Drawing for the job (mm, zero at the part's lowest x, y, z). A direction names the side the tool comes from. Coordinates: 2 decimals unless noted, no trailing zeros. Write each loop counter-clockwise with the first axis right and the second up, starting at its lowest first coordinate (ties: lowest second). Pieces come first, ordered by that corner, then holes. Notation, with made-up numbers: (12.25, -33) -> (70.25, -33) arc R22 cw to (70.25, -13) -> close; hole circle Ø6 at (41.5, 72). An arc over 180 degrees is marked (long way). Write item = value, one per line. Start each with the question number.
Q1. Pull direction X, two halves, no side cores. Call the marked faces 1, 2 and 3: released by +X, released by -X, zero draft, split by the parting line, or undercut.
Q2. Probe line 1 (X direction, y = 11, z = 28); line 2 (Y direction, x = 8.5, z = 26.5); line 3 (Y direction, x = 5.25, z = 4.5). List the from-to ranges inside material, lowest first.
Q3. Band-saw the part on C-C, the plane x = 5.75. List the corners of the cut face in (y, z).
Q4. Band-saw the part on A-A, the plane z = 15. List the corners of the cut face in (x, y), plus the area to 3 significant figures.
Q5. Tool access for the marked faces 4 and 5: list every direction of +Z, -Z, +X, -X, +Y, -Y with a clear straight run to the whole face (end or side of a thin tool).
Q6. Pin check, flat tips, straight feed: P1, Ø1.5, axis at x = 5.5, z = 5, coming from the -Y side; P2, Ø1.5, axis at x = 8, y = 8.5, coming from the -Z side; P3, Ø1.5, axis at x = 5.5, y = 11, coming from the +Z side. Stop position of each tip, or through.
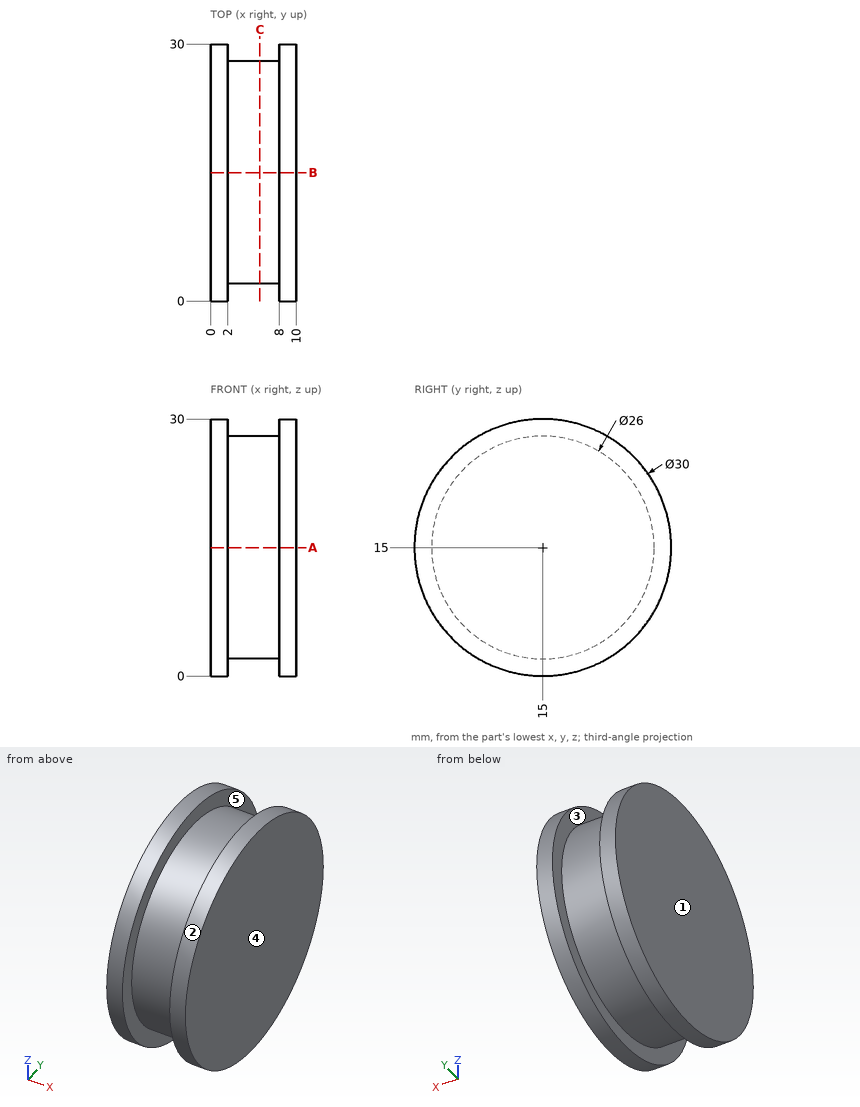
Ans:
q1.face_1 = released by -X
q1.face_2 = zero draft
q1.face_3 = undercut
q2.line_1 = 0 to 2, 8 to 10
q2.line_2 = 5.37 to 24.63
q2.line_3 = 7.34 to 22.66
q3.outline = circle Ø26 at (15, 15)
q4.outline = (0, 0) -> (2, 0) -> (2, 2) -> (8, 2) -> (8, 0) -> (10, 0) -> (10, 30) -> (8, 30) -> (8, 28) -> (2, 28) -> (2, 30) -> (0, 30) -> close
q4.area = 276 mm2
q5.face_4 = +Z, -Z, +X, +Y, -Y
q5.face_5 = none
q6.P1 = 5.87
q6.P2 = 1.15
q6.P3 = 27.59
